Verification items for the finished model (mm, model axes). Face numbers are marked on the shaded views. A direction names the side the tool comes from. Give positions to 0.01 mm unless a question says otherwise; leave off trailing zeros. Order: outer loops, then holes, each group sorted by start corner. A loop starts at its lowest first (then second) coordinate and runs counter-clockwise, first axis right, second up. Notation, with made-up numbers: M 60.5,51 L 119.5,51 A28 ccw 119.5,86 Z; hole C 8,-16.75 d4. An arc over 180 degrees is marked long. Answer as a JSON object with one key per item and string values.
```python
from build123d import *

# Parameters (mm, degrees)
SKETCH_2_R = 2


with BuildPart() as part:
    # Эскиз1 → Повернуть1 (revolve)
    with BuildSketch(Plane.XY, mode=Mode.PRIVATE) as revolve_1_sk:
        Polygon((-2.231746032, 0), (-21.231746032, 0), (-21.231746032, 5.5), (-14.231746032, 5.5), (-14.231746032, 5.25), (-12.231746032, 5.25), (-12.231746032, 6.25), (-10.731746032, 6.25), (-10.731746032, 5), (-2.231746032, 5), align=None)
    revolve(revolve_1_sk.sketch.rotate(Axis((-2.231746032, 0, 0), (-1, 0, 0)), 90), axis=Axis((-2.231746032, 0, 0), (-1, 0, 0)))

    # Эскиз2 → Вырез-Повернуть2 (revolve, cut)
    with BuildSketch(Plane.XY, mode=Mode.PRIVATE) as cut_revolve_2_sk:
        with Locations((-16.731746032, 5.5)):
            Circle(SKETCH_2_R)
        with BuildLine():
            Line((-2.231746032, 0), (-21.231746032, 0))
            Line((-21.231746032, 0), (-21.231746032, 5.039277614))
            ThreePointArc((-21.231746032, 5.039277614), (-18.822332125, 4.058469356), (-17.231746032, 2))
            Line((-17.231746032, 2), (-15.608822853, 2))
            Line((-15.608822853, 2), (-15.231746032, 2.518837092))
            Line((-15.231746032, 2.518837092), (-2.231746032, 4))
            Line((-2.231746032, 4), (-2.231746032, 0))
        make_face()
    revolve(cut_revolve_2_sk.sketch.rotate(Axis((-2.231746032, 0, 0), (-1, 0, 0)), 90), axis=Axis((-2.231746032, 0, 0), (-1, 0, 0)), mode=Mode.SUBTRACT)


solid = part.part
```
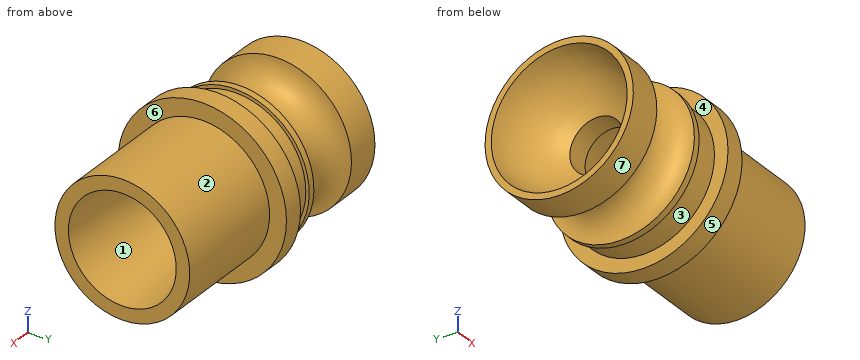
Q1. Gauge pin test, flat ends, axial feed: pin 1 Ø3 at (y, z) = (0, 0) entering from -X; pin 2 Ø5 at (x, z) = (-12.5, -0.5) entering from +Y; pin 3 Ø3 at (x, z) = (-13, 3) entering from -Y; pin 4 Ø1.5 at (y, z) = (2, 1) entering from -X. Record the tip position at first contact, or that the pin passes through.
Resolved:
{"pin 1": "passes through", "pin 2": "stops at y = 6.25", "pin 3": "stops at y = -6.01", "pin 4": "stops at x = -17.78"}
Q2. Tool access check on the marked faces 5, 6 and 7. Record the directions out of +Z, -Z, +X, -X, +Y, -Y that give a thin tool (end or side, any length) a straight path to the whole face; none if there is none.
Resolved:
{"face 5": "+X, -X", "face 6": "+X", "face 7": "-X"}
Q3. Material ranges on L1, parallel to X at y = -4, z = 3.5; L2, parallel to Y at x = -16, z = 0; L3, parallel to Y at x = -16.5, z = 0, recorded low to high.
Resolved:
{"L1": "x = -21.23 to -18.72, -14.74 to -14.23, -12.23 to -10.73", "L2": "y = -3.64 to -2, 2 to 3.64", "L3": "y = -3.51 to -2, 2 to 3.51"}
Q4. Section check A-A on x = -13.25. Record the cut outline in (y, z).
Resolved:
{"outline": "C 0,0 d10.5; hole C 0,0 d5.49"}
Q5. Release check for a two-part mould opening along X. For the marked faces 1, 2, 3 and 4 record: +X half, -X half, draft (parallel to the pull), parting line (faces both ways), or undercut.
Resolved:
{"face 1": "+X half", "face 2": "draft", "face 3": "undercut", "face 4": "undercut"}
